```python
from build123d import *

# Parameters (mm, degrees)
SKETCH1_W           = 50
SKETCH1_H           = 50
BOSS_EXTRUDE1_DEPTH = 3.175
SKETCH2_W           = 3.175
SKETCH2_H           = 33.02
SKETCH2_W_2         = 33.02
SKETCH2_H_2         = 3.18
CUT_EXTRUDE1_DEPTH  = 36.497614356
SKETCH3_R           = 1.6
CUT_EXTRUDE2_DEPTH  = 36.497614356
FILLET1_R           = 10


with BuildPart() as part:
    # Sketch1 → Boss-Extrude1 (new body)
    with BuildSketch(Plane(origin=(0, 0, 0), x_dir=(1, 0, 0), z_dir=(0, 1, 0))):
        Rectangle(SKETCH1_W, SKETCH1_H)
    extrude(amount=BOSS_EXTRUDE1_DEPTH)

    # Sketch2 → Cut-Extrude1 (cut, through all)
    with BuildSketch(Plane(origin=(0, 3.175, 0), x_dir=(1, 0, 0), z_dir=(0, 1, 0))):
        with Locations((19.0945, -0.108)):
            Rectangle(SKETCH2_W, SKETCH2_H)
        with Locations((-4.21, -19.09)):
            Rectangle(SKETCH2_W_2, SKETCH2_H_2)
    extrude(amount=-CUT_EXTRUDE1_DEPTH, mode=Mode.SUBTRACT)

    # Sketch3 → Cut-Extrude2 (cut, through all)
    with BuildSketch(Plane(origin=(0, 3.175, 0), x_dir=(1, 0, 0), z_dir=(0, 1, 0))):
        with Locations(Location((-7.071067812, 17.928932188, 0), (0, 0, 270))):
            Circle(SKETCH3_R)
        with Locations(Location((-17.928932188, 7.071067812, 0), (0, 0, 270))):
            Circle(SKETCH3_R)
    extrude(amount=-CUT_EXTRUDE2_DEPTH, mode=Mode.SUBTRACT)

    # Fillet1
    fillet1_edges = [part.edges().sort_by_distance(p)[0] for p in [
        (25, 1.5875, 25),
        (-25, 1.5875, 25),
        (-25, 1.5875, -25),
        (25, 1.5875, -25),
    ]]
    fillet(fillet1_edges, radius=FILLET1_R)


solid = part.part
```
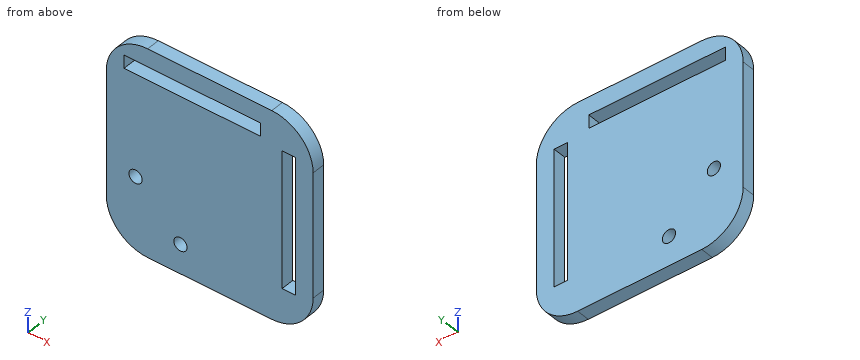
Geometry: final body of the model. Coordinates: model frame, mm. Round coordinates to 2 decimals unless told otherwise and drop trailing zeros. Order: outer loops, then holes, each group sorted by start corner. A loop starts at its lowest first (then second) coordinate and runs counter-clockwise, first axis right, second up. Notation, with made-up numbers: (37, 10.25) - (62, 10.25) arc R35 ccw to (62, 43.25) - close; hole circle Ø1 at (82, 87). An arc over 180 degrees is marked (long way). Write item = value, one per line. Start each with the question number.
Q1. Cut plane A-A on x = -3. Return the cut outline in (y, z) (3 decimals), and give its area (3 significant figures).
Q2. Cut plane C-C on y = 2. Return the cut outline in (x, z), and give its area (3 significant figures).
Q3. Cut plane B-B on z = -11. Return the cut outline in (x, y) (3 decimals).
Q4. Ray query, line 1 (X direction, y = 2.65, z = -13.5); line 2 (Z direction, x = 0.5, y = 1.15); line 3 (Z direction, x = -18.5, y = 2.15). Return the intervals inside material, ascending. Write a range as from..to.
Q5. Pin query (flat end, axial travel): pin 1 (1.6 mm diameter, centred on y = 1.5, z = 19.5, fed in from +X); pin 2 (1 mm diameter, centred on x = 19.5, y = 2, fed in from -Z). Return the tip coordinate at first contact, or that it passes through.
Outcome:
q1.outline = (0, -25) - (3.175, -25) - (3.175, 17.5) - (0, 17.5) - close; (0, 20.68) - (3.175, 20.68) - (3.175, 25) - (0, 25) - close
q1.area = 149 mm^2
q2.outline = (-25, -15) arc R10 ccw to (-15, -25) - (15, -25) arc R10 ccw to (25, -15) - (25, 15) arc R10 ccw to (15, 25) - (-15, 25) arc R10 ccw to (-25, 15) - close; hole (-20.72, 17.5) - (12.3, 17.5) - (12.3, 20.68) - (-20.72, 20.68) - close; hole circle Ø3.2 at (-17.93, -7.07); hole circle Ø3.2 at (-7.07, -17.93); hole (17.51, -16.4) - (20.68, -16.4) - (20.68, 16.62) - (17.51, 16.62) - close
q2.area = 2,190 mm^2
q3.outline = (-25, 0) - (17.507, 0) - (17.507, 3.175) - (-25, 3.175) - close; (20.682, 0) - (25, 0) - (25, 3.175) - (20.682, 3.175) - close
q4.line_1 = -25..17.51, 20.68..25
q4.line_2 = -25..17.5, 20.68..25
q4.line_3 = -24.37..-8.57, -5.58..17.5, 20.68..24.37
q5.pin_1 = 24.29
q5.pin_2 = -24.17
